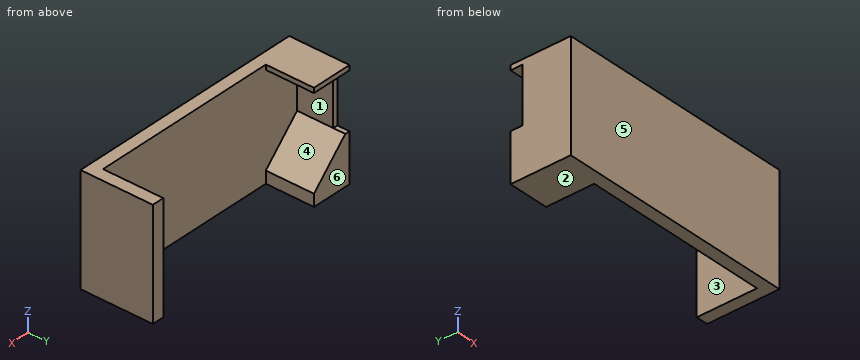
from build123d import *

# Parameters (mm, degrees)
SKETCH1_W           = 5
SKETCH1_H           = 45
SKETCH1_W_2         = 2
SKETCH1_H_2         = 23
SKETCH1_W_3         = 15
SKETCH1_H_3         = 2
BOSS_EXTRUDE1_DEPTH = 5
SKETCH1_4_W         = 5
SKETCH1_4_H         = 45
BOSS_EXTRUDE2_DEPTH = 25
SKETCH1_5_W         = 15
SKETCH1_5_H         = 2
SKETCH1_5_W_2       = 2
BOSS_EXTRUDE3_DEPTH = 20
BOSS_EXTRUDE4_DEPTH = 20
SKETCH1_8_W         = 2
SKETCH1_8_H         = 23
BOSS_EXTRUDE5_DEPTH = 15


with BuildPart() as part:
    # Sketch1 → Boss-Extrude1 (new body)
    with BuildSketch(Plane(origin=(0, 0, 0), x_dir=(1, 0, 0), z_dir=(0, 1, 0))):
        Polygon((-50, 2.5), (-48, 2.5), (-33, 17.5), (-33, 22.5), (-50, 22.5), align=None)
        Polygon((-48, 2.5), (-48, -20.5), (-33, -20.5), (-33, -22.5), (45, -22.5), (45, 22.5), (-28, 22.5), (-33, 17.5), align=None)
        Polygon((-33, 22.5), (-33, 17.5), (-28, 22.5), align=None)
        with Locations((47.5, 0)):
            Rectangle(SKETCH1_W, SKETCH1_H)
        with Locations((-49, -9)):
            Rectangle(SKETCH1_W_2, SKETCH1_H_2)
        with Locations((-40.5, -21.5)):
            Rectangle(SKETCH1_W_3, SKETCH1_H_3)
        with Locations((-49, -21.5)):
            Rectangle(SKETCH1_W_2, SKETCH1_H_3)
    extrude(amount=-BOSS_EXTRUDE1_DEPTH)

    # Sketch1_4 → Boss-Extrude2 (add)
    with BuildSketch(Plane(origin=(0, 0, 0), x_dir=(1, 0, 0), z_dir=(0, 1, 0))):
        with Locations((47.5, 0)):
            Rectangle(SKETCH1_4_W, SKETCH1_4_H)
    extrude(amount=BOSS_EXTRUDE2_DEPTH)

    # Sketch1_5 → Boss-Extrude3 (add)
    with BuildSketch(Plane(origin=(0, 0, 0), x_dir=(1, 0, 0), z_dir=(0, 1, 0))):
        with Locations((-40.5, -21.5)):
            Rectangle(SKETCH1_5_W, SKETCH1_5_H)
        with Locations((-49, -21.5)):
            Rectangle(SKETCH1_5_W_2, SKETCH1_5_H)
    extrude(amount=BOSS_EXTRUDE3_DEPTH)

    # Sketch1_6 → Boss-Extrude4 (add)
    with BuildSketch(Plane(origin=(0, 0, 0), x_dir=(1, 0, 0), z_dir=(0, 1, 0))):
        Polygon((-50, 2.5), (-48, 2.5), (-33, 17.5), (-33, 22.5), (-50, 22.5), align=None)
    extrude(amount=BOSS_EXTRUDE4_DEPTH)

    # Sketch1_8 → Boss-Extrude5 (add)
    with BuildSketch(Plane(origin=(0, 0, 0), x_dir=(1, 0, 0), z_dir=(0, 1, 0))):
        with Locations((-49, -9)):
            Rectangle(SKETCH1_8_W, SKETCH1_8_H)
    extrude(amount=BOSS_EXTRUDE5_DEPTH)


solid = part.part
Build history of the part. All positions in model axes, mm. Face numbers are marked on the shaded views. A direction names the side the tool comes from. Round coordinates to 2 decimals unless told otherwise and drop trailing zeros. Order: outer loops, then holes, each group sorted by start corner. A loop starts at its lowest first (then second) coordinate and runs counter-clockwise, first axis right, second up. Notation, with made-up numbers: M 17,46 L 37,46 A24 cw 37,71 Z; hole C -6,-5 d2. An arc over 180 degrees is marked long. Use CSV: the item, a comma, the result in double quotes. Start each with the question number.
(1) Cut at B-B on z = -14. List the corners of the cut face in (x, y), then the cut area to 3 significant figures.
(2) Cut at A-A on y = 3.25. List the corners of the cut face in (x, z), then the cut area to 4 significant figures.
(3) Cut at D-D on x = -26.5. List the corners of the cut face in (y, z).
(4) Tool access for the marked faces 4, 5 and 6: list every direction of +Z, -Z, +X, -X, +Y, -Y with a clear straight run to the whole face (end or side of a thin tool).
(5) Drill centre lines: probe 1 along Y at (x, z) = (-18, -16); probe 2 along X at (y, z) = (22.75, -11.5); probe 3 along X at (y, z) = (18.5, -9.5). Where is each one in solid material? Low to high.
(6) Cut at C-C on x = -39. List the corners of the cut face in (y, z).
(7) Flat gauge pins, fed straight in: P1, Ø8.5, axis at x = -40.5, z = -8.5, coming from the +Y side; P2, Ø13.5, axis at x = 0, z = 8.5, coming from the +Y side; P3, Ø1, axis at x = -49, z = 7.5, coming from the +Y side. Where does each tip first touch, or does it go through?
(8) Mould opens along Z. For the marked faces 1, 2 and 3 say: +Z half, -Z half, draft (parallel to the pull), parting line (faces both ways), or undercut.
Findings:
1,outline,"M -50,-5 L 50,-5 L 50,25 L 45,25 L 45,0 L -36.5,0 L -36.5,20 L -50,20 Z"
1,area,"895 mm^2"
2,outline,"M -50,-22.5 L -33,-22.5 L -33,-17.5 L -48,-2.5 L -48,20.5 L -33,20.5 L -33,22.5 L -50,22.5 Z; M 45,-22.5 L 50,-22.5 L 50,22.5 L 45,22.5 Z"
2,area,"532.5 mm^2"
3,outline,"M -5,-22.5 L 0,-22.5 L 0,22.5 L -5,22.5 Z"
4,face 4,"+Y"
4,face 5,"+Z, -Z, +X, -X, -Y"
4,face 6,"+Z, -Z, -X, +Y"
5,probe 1,"y = -5 to 0"
5,probe 2,"x = 45 to 50"
5,probe 3,"x = -50 to -41, 45 to 50"
6,outline,"M -5,-22.5 L 20,-22.5 L 20,-11.5 L 0,-11.5 L 0,20.5 L 20,20.5 L 20,22.5 L -5,22.5 Z"
7,P1,"stops at y = 20"
7,P2,"stops at y = 0"
7,P3,"stops at y = 15"
8,face 1,"undercut"
8,face 2,"-Z half"
8,face 3,"draft"
